Drawing for the job (mm, zero at the part's lowest x, y, z). Coordinates: 2 decimals unless noted, no trailing zeros. Write each loop counter-clockwise with the first axis right and the second up, starting at its lowest first coordinate (ties: lowest second). Pieces come first, ordered by that corner, then holes. Notation, with made-up numbers: (71, 60.25) -> (79, 60.25) arc R23 ccw to (79, 93.25) -> close; hole circle Ø1 at (-2, 75). An arc over 180 degrees is marked (long way). Answer as CSV lines item,"result". Start each with the question number.
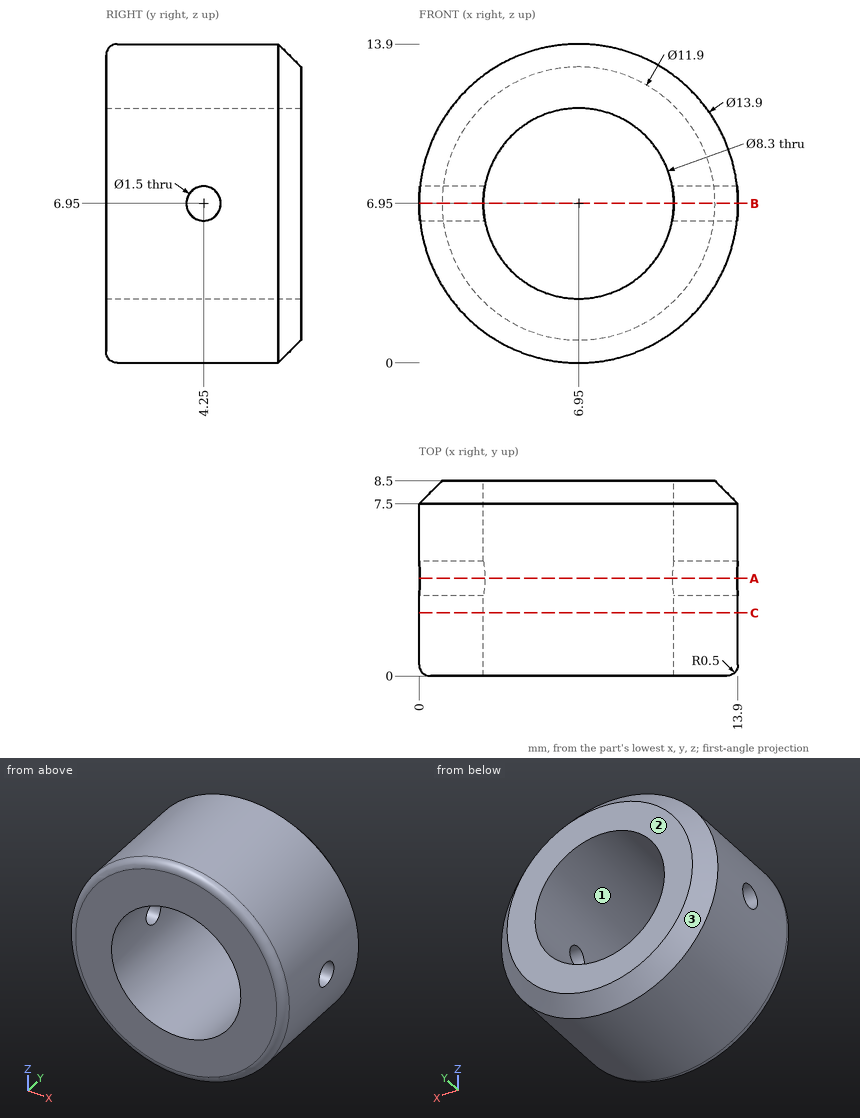
1. Cut at B-B (z = 6.95). Count the separate pieces of the cut face and the enclosed holes in it, then the cut area to 3 significant figures.
2. Mould opens along Z. For the marked faces 1, 2 and 3 say: pulls with the +Z half, pulls with the -Z half, needs draft (parallel to the pull), parting line crosses it, or undercut.
3. Cut at A-A (y = 4.25). Give the cut face in (x, z), then the cut area to 3 significant figures.
4. Cut at C-C (y = 2.75). Give the cut face in (x, z), then the cut area to 3 significant figures.
5. Wall check: line 1 (X direction, y = 5.5, z = 6.95); line 2 (Y direction, x = 1.6, z = 6.95); line 3 (X direction, y = 6, z = 8.25). Give the ranges that are in metal, low to high.
6. Flat gauge pins, fed straight in: P1, Ø3, axis at y = 1.5, z = 3, coming from the +X side; P2, Ø6.5, axis at x = 6.95, z = 6.95, coming from the +Y side; P3, Ø1.5, axis at y = 3.5, z = 8.5, coming from the -X side. Where does each tip first touch, or does it go through?
Geometry check:
1,separate pieces,"4"
1,enclosed holes,"0"
1,area,"38.1 mm²"
2,face 1,"undercut"
2,face 2,"needs draft"
2,face 3,"parting line crosses it"
3,outline,"(0.04, 6.2) arc R6.95 ccw to (13.86, 6.2) -> (11.03, 6.2) arc R4.15 cw to (2.87, 6.2) -> close; (0.04, 7.7) -> (2.87, 7.7) arc R4.15 cw to (11.03, 7.7) -> (13.86, 7.7) arc R6.95 ccw to start"
3,area,"89.2 mm²"
4,outline,"circle Ø13.9 at (6.95, 6.95); hole circle Ø8.3 at (6.95, 6.95)"
4,area,"97.6 mm²"
5,line 1,"0 to 2.8, 11.1 to 13.9"
5,line 2,"0 to 3.5, 5 to 8.5"
5,line 3,"0.12 to 3.01, 10.89 to 13.78"
6,P1,"x = 13.45"
6,P2,"through"
6,P3,"x = 0.05"
